Geometry check sheet. Reference: the model listing, model coordinates, mm. Face numbers are marked on the shaded views. A direction names the side the tool comes from. Give positions to 0.01 mm unless a question says otherwise; leave off trailing zeros. Loops run counter-clockwise (first coordinate to the right, second up) from the corner with the lowest first, then second, coordinate; pieces in that order, holes last.
1. Release check for a two-part mould opening along Y. For the marked faces 1, 2, 3 and 4 record: +Y half, -Y half, draft (parallel to the pull), parting line (faces both ways), or undercut.
2. Cross-section at D-D, the plane z = -2.75. Record the cut outline in (x, y), plus the area to 3 significant figures.
3. Cross-section at A-A, the plane z = -7.25. Record the cut outline in (x, y), plus the area to 3 significant figures.
4. Tool access check on the marked faces 5, 6 and 7. Record the directions out of +Z, -Z, +X, -X, +Y, -Y that give a thin tool (end or side, any length) a straight path to the whole face; none if there is none.
5. Go/stop test with flat-tipped pins: pin 1 Ø1.3 at (y, z) = (0.5, -12) entering from -X; pin 2 Ø1.3 at (x, z) = (12, -7) entering from -Y; pin 3 Ø6 at (x, z) = (2, -8.5) entering from +Y. Record where each tip stops, or that it passes through.
6. Material ranges on L1, parallel to Y at x = 0.5, z = -2.25; L2, parallel to X at y = 6.5, z = -1; L3, parallel to Z at x = 11.5, y = 6, recorded low to high.
7. Cross-section at B-B, the plane x = 4.75. Record the cut outline in (y, z), plus the area to 3 significant figures.
8. Cross-section at C-C, the plane y = 8.75. Record the cut outline in (x, z), plus the area to 3 significant figures.
Autodesk Inventor part; units mm, degrees
ref_plane "Flange Pattern Plane" through (12.7, 7.9375, -4.5466) normal (0, 1, 0) x (1, 0, 0)
ref_plane "YZ Plane" through (0, 0, 0) normal (1, 0, 0) x (0, 1, 0)
ref_plane "XZ Plane" through (0, 0, 0) normal (0, 1, 0) x (-1, 0, 0)
sketch "Sketch1" plane through (0, 0, 0) normal (0, 1, 0) x (-1, 0, 0)
  line L0 (-12.7, 0) -> (12.7, 0)
  line L1 (12.7, 0) -> (12.7, -12.7)
  line L2 (12.7, -12.7) -> (-12.7, -12.7)
  line L3 (-12.7, -12.7) -> (-12.7, 0)
  line L4 (12.7, 0) -> (-12.7, -12.7) construction
  point P0 (0, 0)
  point P1 (0, 0)
  dimension "d0" = 25.4
  dimension "d1" = 12.7
extrude "Plate1" add sketch "Sketch1" along normal blind 1.5875
sketch "Sketch2" plane through (11.1125, 0, -12.7) normal (1, 0, 0) x (0, 1, 0)
  line L0 (0, 12.7) -> (0, 0)
  line L1 (0, 0) -> (14.2875, 0)
  line L2 (14.2875, 0) -> (14.2875, 12.7)
  line L3 (14.2875, 12.7) -> (0, 12.7)
edge flange "Flanges" height 12.7 angle 90 thickness 1.5875 bend radius 0.7937 thickness toward (1, 0, 0) relief tear relief width 1.5875 relief depth 0.7937 corner gap 1.5875 corner form 0 edges at (12.7, 1.5875, -6.35) (-12.7, 1.5875, -6.35) wall of the first edge with corners at (11.1125, 0, 0) (11.1125, 0, -12.7) (11.1125, 14.2875, -12.7) (11.1125, 14.2875, 0)
bend "Bend1"
corner "Corner1"
sketch "Sketch3" plane through (12.7, 2.3812, -12.7) normal (1, 0, 0) x (0, 0, -1)
  line L0 (-8.1534, 7.8676) -> (-4.5466, 7.8676)
  line L1 (-4.0386, 7.3596) -> (-4.0386, 3.7528)
  line L2 (-4.5466, 3.2448) -> (-8.1534, 3.2448)
  line L3 (-8.6614, 3.7528) -> (-8.6614, 7.3596)
  arc A0 (-8.1534, 7.8676) -> (-8.6614, 7.3596) centre (-8.1534, 7.3596) ccw
  arc A1 (-4.0386, 7.3596) -> (-4.5466, 7.8676) centre (-4.5466, 7.3596) ccw
  arc A2 (-4.5466, 3.2448) -> (-4.0386, 3.7528) centre (-4.5466, 3.7528) ccw
  arc A3 (-8.6614, 3.7528) -> (-8.1534, 3.2448) centre (-8.1534, 3.7528) ccw
  line L4 (-12.7, 0) -> (-12.7, 11.9062) construction
  line L5 (-12.7, 11.9062) -> (0, 11.9062) construction
  line L6 (-8.1534, 7.3596) -> (-4.5466, 3.7528) construction
  point P0 (-12.7, -2.3813)
  point P1 (-4.0386, 3.2448)
  point P2 (-8.6614, 3.2448)
  point P3 (-6.35, 5.5562)
  dimension "d16" = 4.6228
  dimension "d17" = 0.508
  dimension "d20" = 6.35
  dimension "d21" = 6.35
extrude "Flange Stamp" cut sketch "Sketch3" against normal blind 1.5875
sketch "Sketch7" plane through (12.7, 2.3813, 0) normal (1, 0, 0) x (0, 0, -1)
  arc A0 (4.5466, 7.8676) -> (4.0386, 7.3596) centre (4.5466, 7.3596) ccw construction
  arc A1 (8.1534, 3.2448) -> (8.6614, 3.7528) centre (8.1534, 3.7528) ccw construction
  circle A2 centre (6.35, 5.5563) radius 2.1844
  line L0 (4.5466, 7.3596) -> (8.1534, 3.7528) construction
  point P0 (0, -2.3813)
  dimension "d46" = 4.3688
surface extrude "Flange Circle" sketch "Sketch7" against normal up to surface (1.5875 mm away) shown yes curves A2
ref_plane "Flange Pattern Plane" through (12.7, 7.9375, -4.5466) normal (0, 1, 0) x (1, 0, 0)
sketch "Flange Pattern Sketch" plane through (12.7, 7.9375, -4.5466) normal (0, 1, 0) x (1, 0, 0)
  line L0 (0, 3.6068) -> (0, 0) construction
  line L1 (-30.5786, -4.5466) -> (5.6718, -4.5466) construction
  line L2 (0, 0) -> (-1.5875, 0) construction
  point P0 (-12.7, -4.5466)
  point P1 (0, 1.8034)
  point P2 (0, 14.5034)
  dimension "d43" = 25.4
  dimension "d40" = 12.7
feature "Flange Pattern" [suppressed]
sketch "Sketch8" plane through (0, 0, 0) normal (0, -1, 0) x (1, 0, 0)
  line L0 (10.3187, 0) -> (-10.3187, 0) construction
  line L1 (8.1534, -4.0386) -> (4.5466, -4.0386)
  line L2 (4.0386, -4.5466) -> (4.0386, -8.1534)
  line L3 (4.5466, -8.6614) -> (8.1534, -8.6614)
  line L4 (8.6614, -8.1534) -> (8.6614, -4.5466)
  arc A0 (8.6614, -4.5466) -> (8.1534, -4.0386) centre (8.1534, -4.5466) ccw
  arc A1 (8.1534, -8.6614) -> (8.6614, -8.1534) centre (8.1534, -8.1534) ccw
  arc A2 (4.0386, -8.1534) -> (4.5466, -8.6614) centre (4.5466, -8.1534) ccw
  arc A3 (4.5466, -4.0386) -> (4.0386, -4.5466) centre (4.5466, -4.5466) ccw
  line L5 (8.1534, -4.5466) -> (4.5466, -8.1534) construction
  line L6 (12.7, 0) -> (12.7, -12.7) construction
  point P0 (0, 0)
  point P1 (4.0386, -8.6614)
  point P2 (8.6614, -8.6614)
  point P3 (6.35, -6.35)
  dimension "d49" = 4.6228
  dimension "d50" = 0.508
  dimension "d51" = 6.35
  dimension "d52" = 6.35
extrude "Body Stamp" cut sketch "Sketch8" against normal blind 1.5875
sketch "Sketch9" plane through (0, 0, 0) normal (0, -1, 0) x (1, 0, 0)
  arc A0 (8.6614, -4.5466) -> (8.1534, -4.0386) centre (8.1534, -4.5466) ccw construction
  arc A1 (4.0386, -8.1534) -> (4.5466, -8.6614) centre (4.5466, -8.1534) ccw construction
  line L0 (8.1534, -4.5466) -> (4.5466, -8.1534) construction
  circle A2 centre (6.35, -6.35) radius 2.1844
  point P0 (0, 0)
  dimension "d55" = 4.3688
surface extrude "Body Circle" sketch "Sketch9" against normal up to surface (1.5875 mm away) shown yes curves A2
sketch "Body Pattern Sketch" plane through (0, 0, 0) normal (0, -1, 0) x (1, 0, 0)
  line L0 (10.3187, 0) -> (-10.3187, 0) construction
  line L1 (12.7, 0) -> (12.7, -12.7) construction
  point P0 (0, 0)
  point P1 (6.35, -6.35)
  point P2 (6.35, -19.05)
  dimension "d62" = 12.7
  dimension "d65" = 12.7
  dimension "d58" = 6.35
  dimension "d99" = 6.35
feature "Body Pattern" [suppressed]
sketch "Sketch15" plane through (0, 0, 0) normal (0, -1, 0) x (1, 0, 0)
  line L0 (10.3187, 0) -> (-10.3187, 0) construction
  line L1 (1.8034, -10.3886) -> (-1.8034, -10.3886)
  line L2 (-2.3114, -10.8966) -> (-2.3114, -14.5034)
  line L3 (-1.8034, -15.0114) -> (1.8034, -15.0114)
  line L4 (2.3114, -14.5034) -> (2.3114, -10.8966)
  arc A0 (2.3114, -10.8966) -> (1.8034, -10.3886) centre (1.8034, -10.8966) ccw
  arc A1 (1.8034, -15.0114) -> (2.3114, -14.5034) centre (1.8034, -14.5034) ccw
  arc A2 (-1.8034, -10.3886) -> (-2.3114, -10.8966) centre (-1.8034, -10.8966) ccw
  arc A3 (-2.3114, -14.5034) -> (-1.8034, -15.0114) centre (-1.8034, -14.5034) ccw
  line L5 (1.8034, -10.8966) -> (-1.8034, -14.5034) construction
  line L6 (12.7, 0) -> (12.7, -12.7) construction
  point P0 (0, 0)
  point P1 (-2.3114, -15.0114)
  point P2 (2.3114, -15.0114)
  point P3 (0, -12.7)
  dimension "d106" = 4.6228
  dimension "d107" = 0.508
  dimension "d108" = 12.7
  dimension "d109" = 12.7
extrude "Center Stamp" cut sketch "Sketch15" against normal blind 1.5875
extrude_surface "Center Circle" [suppressed]
pattern_linear "Center Pattern" [suppressed]
sketch "Arc Length" plane through (11.1125, 2.3813, 0) normal (0, 0, 1) x (1, 0, 0)
  line L0 (0, 0) -> (1.5875, 0) construction
  arc A0 (-0.7937, -0.7938) -> (0, 0) centre (-0.7937, 0) ccw construction
  line L1 (-0.7937, -2.3813) -> (-0.7937, -0.7938) construction
  arc A1 (-0.7937, -2.3813) -> (1.5875, 0) centre (-0.7937, 0) ccw construction
  point P0 (-11.1125, -2.3813)
  dimension "d85" = 3.7405
  dimension "d92" = 1.2468
feature "Notch" [suppressed]
mirror "Notch Mirror" [suppressed]
pattern_linear "Notch Pattern" [suppressed]
chamfer "End Chamfer" distance 1.016 angle 45 4 edges at (-11.9062, 14.2875, -12.7) (11.9063, 14.2875, -12.7) (-11.9062, 14.2875, 0) (11.9062, 14.2875, 0)
sketch "Sketch14" plane through (-12.7, 2.3813, 431.8) normal (1, 0, 0) x (0, 0, -1)
  line L0 (431.8, 11.9063) -> (444.5, 11.9063) construction
  line L1 (431.8, 0) -> (431.8, 11.9063) construction
  line L2 (431.8, -2.3813) -> (444.5, -2.3813) construction
  line L3 (431.8, 11.9063) -> (444.5, 11.9063)
  line L4 (444.5, 11.9063) -> (444.5, -2.3813)
  line L5 (444.5, -2.3813) -> (431.8, -2.3813)
  line L6 (431.8, -2.3813) -> (431.8, 11.9063)
  point P0 (62.4078, 11.9062)
  point P1 (432.816, 11.9063)
  point P2 (431.8, 10.8903)
  point P3 (431.8, -2.3812)
  point P4 (382.0521, -1.9844)
  point P5 (443.484, 11.9063)
  point P6 (254.9398, 11.9062)
  point P7 (316.4078, 11.9062)
extrude "Half Cut" cut sketch "Sketch14" along normal blind 12.7
sketch "Sketch13" plane through (12.7, 14.2875, 0) normal (1, 0, 0) x (0, 0, -1)
  line L0 (0, 0) -> (12.7, 0) construction
  line L1 (62.4078, 0) -> (63.4238, -1.016)
  line L2 (63.4238, -1.016) -> (64.4398, 0)
  line L3 (62.4078, 0) -> (64.4398, 0)
  line L4 (12.7, -11.9062) -> (0, -11.9062) construction
  line L5 (63.4238, -10.8903) -> (61.161, -13.1531)
  line L6 (61.161, -13.1531) -> (63.4238, -15.4159)
  line L7 (63.4238, -15.4159) -> (65.6866, -13.1531)
  line L8 (65.6866, -13.1531) -> (63.4238, -10.8903)
  line L9 (63.4238, -10.8903) -> (63.4238, -15.4159) construction
  line L10 (63.4238, -1.016) -> (63.4238, -10.8903) construction
  line L11 (0, -11.9062) -> (12.7, -11.9062) construction
  point P0 (0, -14.2875)
  dimension "d86" = 4.5256
  dimension "d88" = 1.016
  dimension "d91" = 1.016
  dimension "d102" = 63.4238
sketch "Sketch16" plane through (0, 0, 0) normal (0, -1, 0) x (1, 0, 0)
  circle A0 centre (0, -12.7) radius 2.1844
  line L0 (10.3187, 0) -> (-10.3187, 0) construction
  line L1 (12.7, 0) -> (12.7, -12.7) construction
  point P0 (0, 0)
  dimension "d112" = 4.3688
  dimension "d118" = 12.7
  dimension "d119" = 12.7
equation "\"d18\" = Thickness"
equation "\"d53\" = Thickness"
equation "\"d89\" = Thickness"
equation "\"d1\" = 1.27 * Length"
equation "\"d2\" = Thickness"
equation "\"d3\" = BendReliefWidth"
equation "\"d4\" = BendReliefDepth"
equation "\"d5\" = MinimumRemnant"
equation "\"d6\" = TransitionRadius"
equation "\"d10\" = CornerReliefSize"
equation "\"d11\" = GapSize"
equation "\"d12\" = JacobiRadiusSize"
equation "\"BendRadius\" = Thickness"
equation "\"BendReliefWidth\" = Thickness"
equation "\"BendReliefDepth\" = 0.5 * Thickness"
equation "\"CornerReliefSize\" = 4 * Thickness"
equation "\"MinimumRemnant\" = 2 * Thickness"
equation "\"TransitionRadius\" = BendRadius"
equation "\"JacobiRadiusSize\" = BendRadius"
equation "\"GapSize\" = Thickness"
properties part number "Alu C 1x2x1x35"
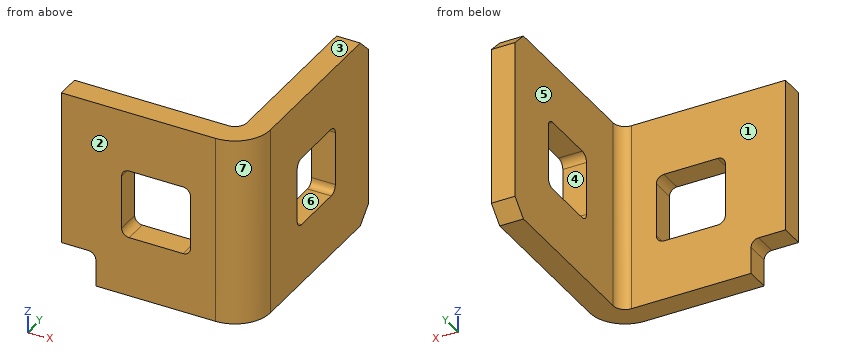
Result:
1. face 1: +Y half
1. face 2: -Y half
1. face 3: draft
1. face 4: undercut
2. outline: (0, 0) - (10.32, 0) arc R2.38 ccw to (12.7, 2.38) - (12.7, 14.29) - (11.11, 14.29) - (11.11, 2.38) arc R0.79 cw to (10.32, 1.59) - (0, 1.59) - close
2. area: 39.2 mm2
3. outline: (0, 0) - (4.04, 0) - (4.04, 1.59) - (0, 1.59) - close; (8.66, 0) - (10.32, 0) arc R2.38 ccw to (12.7, 2.38) - (12.7, 5.63) - (11.11, 5.63) - (11.11, 2.38) arc R0.79 cw to (10.32, 1.59) - (8.66, 1.59) - close; (11.11, 10.25) - (12.7, 10.25) - (12.7, 14.29) - (11.11, 14.29) - close
3. area: 24.6 mm2
4. face 5: +Z, -Z, -X, +Y
4. face 6: +X, -X
4. face 7: +Z, -Z, +X, -Y
5. pin 1: stops at x = 2.31
5. pin 2: stops at y = 0.23
5. pin 3: stops at y = 1.59
6. L1: y = 0 to 1.59
6. L2: x = 11.11 to 12.7
6. L3: z = -12.7 to -8.64, -4.06 to 0
7. outline: (0, -12.7) - (1.59, -12.7) - (1.59, -8.66) - (0, -8.66) - close; (0, -4.04) - (1.59, -4.04) - (1.59, 0) - (0, 0) - close
7. area: 12.8 mm2
8. outline: (11.11, -12.7) - (12.7, -12.7) - (12.7, -8.66) - (11.11, -8.66) - close; (11.11, -4.04) - (12.7, -4.04) - (12.7, 0) - (11.11, 0) - close
8. area: 12.8 mm2
